Could you check a few things on this model? Use its own coordinates, in mm. A direction names the side the tool comes from. Coordinates: 2 decimals unless noted, no trailing zeros. Write each loop counter-clockwise with the first axis right and the second up, starting at its lowest first coordinate (ties: lowest second). Pieces come first, ordered by that corner, then holes. Notation, with made-up numbers: (21.25, 72.25) - (75.25, 72.25) arc R14 cw to (75.25, 94.25) - close; hole circle Ø8 at (4, 29). An arc over 180 degrees is marked (long way). Write item = value, one per line. Start each with the question number.
```python
from build123d import *

# Parameters (mm, degrees)
SKETCH_1_W                 = 50
SKETCH_1_H                 = 6
EXTRUDE_1_DEPTH            = 25
CUT_EXTRUDE_1_REACH        = 57.982
PATTERN_LINEAR_1_COUNT     = 2
PATTERN_LINEAR_1_PITCH     = 10
PATTERN_LINEAR_1_COL_COUNT = 2
PATTERN_LINEAR_1_COL_PITCH = 10


with BuildPart() as part:
    # 草图1 → 凸台-拉伸1 (new, symmetric)
    with BuildSketch(Plane.XY):
        Rectangle(SKETCH_1_W, SKETCH_1_H)
    extrude(amount=EXTRUDE_1_DEPTH, both=True)

    # 草图2 → 切除-拉伸1 (cut, up to next)
    with BuildSketch(Plane.XY.offset(25), mode=Mode.PRIVATE) as cut_extrude_1_sk1:
        with BuildLine():
            Line((-3, -1), (-3, -3))
            Line((-3, -3), (3, -3))
            Line((3, -3), (3, -1))
            ThreePointArc((3, -1), (0, 2), (-3, -1))
        make_face()
    cut_extrude_1_tool1 = extrude(cut_extrude_1_sk1.sketch, amount=-CUT_EXTRUDE_1_REACH, mode=Mode.PRIVATE) & part.part
    cut_extrude_1 = cut_extrude_1_tool1.solids().sort_by_distance((0, -0.770442, 25))[0]
    add(cut_extrude_1, mode=Mode.SUBTRACT)

    # 阵列(线性)1: 切除-拉伸1 ×2
    with Locations(*[(-i * PATTERN_LINEAR_1_PITCH, 0, 0) for i in range(1, PATTERN_LINEAR_1_COUNT)]):
        add(cut_extrude_1, mode=Mode.SUBTRACT)

    # 阵列(线性)1 col: 切除-拉伸1 ×2
    with Locations(*[(i * PATTERN_LINEAR_1_COL_PITCH, 0, 0) for i in range(1, PATTERN_LINEAR_1_COL_COUNT)]):
        add(cut_extrude_1, mode=Mode.SUBTRACT)


solid = part.part
```
1) Thinking about a two-plate mould opening in X: for faces 1 (the cylindrical face through (0, 2, 0)), 2 (the flat face through (-5, -3, 0)), 3 (the flat face through (-25, 0, 0)), which applies, +X half, -X half, draft (parallel to the pull), parting line (faces both ways), or undercut?
2) If I drill on probe 1 along X at (y, z) = (-1, 9); probe 2 along X at (y, z) = (0.35, 13.5); probe 3 along Y at (x, z) = (10, -20), over which ranges is the centre line in solid material (lowest first)? Write a range as [from, to].
3) Suppose I cut it at C-C on x = -10. Please give me the cut outline in (y, z), plus the area to 3 significant figures.
4) Suppose I cut it at B-B on z = 6. Please give me the cut outline in (x, y).
5) Suppose I cut it at A-A on y = -2.05. Please give me the cut outline in (x, z), plus the area to 3 significant figures.
6) Which directions (+Z, -Z, +X, -X, +Y, -Y) give clear straight access to the entire face, cutting with the end or side of a thin tool? Please do faces 4 (the flat face through (-13, -2, 0)), 5 (the flat face through (5, -3, 0)).
Reply:
q1.face_1 = undercut
q1.face_2 = draft
q1.face_3 = -X half
q2.probe_1 = [-25, -13], [-7, -3], [3, 7], [13, 25]
q2.probe_2 = [-25, -12.68], [-7.32, -2.68], [2.68, 7.32], [12.68, 25]
q2.probe_3 = [2, 3]
q3.outline = (2, -25) - (3, -25) - (3, 25) - (2, 25) - close
q3.area = 50.0 mm^2
q4.outline = (-25, -3) - (-13, -3) - (-13, -1) arc R3 cw to (-7, -1) - (-7, -3) - (-3, -3) - (-3, -1) arc R3 cw to (3, -1) - (3, -3) - (7, -3) - (7, -1) arc R3 cw to (13, -1) - (13, -3) - (25, -3) - (25, 3) - (-25, 3) - close
q5.outline = (-25, -25) - (-13, -25) - (-13, 25) - (-25, 25) - close; (-7, -25) - (-3, -25) - (-3, 25) - (-7, 25) - close; (3, -25) - (7, -25) - (7, 25) - (3, 25) - close; (13, -25) - (25, -25) - (25, 25) - (13, 25) - close
q5.area = 1,600 mm^2
q6.face_4 = +Z, -Z, -Y
q6.face_5 = +Z, -Z, +X, -X, -Y
